Read the model definition and answer for the solid it produces. Units are mm, in the model's axes. A direction names the side the tool comes from. Round coordinates to 2 decimals unless told otherwise and drop trailing zeros. Loops run counter-clockwise (first coordinate to the right, second up) from the corner with the lowest first, then second, coordinate; pieces in that order, holes last. Notation, with made-up numbers: M 63.25,72 L 72.25,72 A21 ccw 72.25,91 Z; hole C 75.25,-36.5 d7. An arc over 180 degrees is marked long. Write each question's results on one line, items separated by ' | '.
from build123d import *

# Parameters (mm, degrees)
SKETCH1_R             = 1.5
BOSS_EXTRUDE1_DEPTH   = 5
BOSS_EXTRUDE1_2_DEPTH = 5
SKETCH1_3_R           = 5.25
BOSS_EXTRUDE2_DEPTH   = 2.5
SKETCH1_4_R           = 3.25
BOSS_EXTRUDE3_DEPTH   = 5
CUT_EXTRUDE1_DEPTH    = 34.791042337
CUT_EXTRUDE2_DEPTH    = 34.791042337
LPATTERN1_COUNT       = 28
LPATTERN1_PITCH       = 0.5
CUT_EXTRUDE3_DEPTH    = 34.791042337
CIRPATTERN1_COUNT     = 8
CIRPATTERN1_ANGLE     = 42


with BuildPart() as part:
    # Sketch1 → Boss-Extrude1 (new body)
    with BuildSketch(Plane.XY):
        with BuildLine():
            Line((-1.559459186, 5.819980914), (-9.630372069, 7.89024295))
            ThreePointArc((-9.630372069, 7.89024295), (-13.619847961, 6.086363356), (-12.727105745, 1.8))
            Line((-12.727105745, 1.8), (-9, 1.8))
            Line((-9, 1.8), (-9, 0))
            Line((-9, 0), (-5.25, 0))
            ThreePointArc((-5.25, 0), (-4.165105037, 3.195997502), (-1.358799987, 5.071110588))
            Line((-1.358799987, 5.071110588), (-1.559459186, 5.819980914))
        make_face()
        with Locations((-10.5, 4.5)):
            Circle(SKETCH1_R, mode=Mode.SUBTRACT)
    extrude(amount=BOSS_EXTRUDE1_DEPTH)



with BuildPart() as body_2:
    # Sketch1 → Boss-Extrude1 2 (new body)
    with BuildSketch(Plane.XY):
        with BuildLine():
            Line((5.983025461, -0.728942102), (5.162088265, 0.956736509))
            ThreePointArc((5.162088265, 0.956736509), (4.867715236, -1.966684615), (3.048690517, -4.274106471))
            Line((3.048690517, -4.274106471), (3.844408913, -5.389662519))
            Line((3.844408913, -5.389662519), (13.676957988, -3.567307264))
            Line((13.676957988, -3.567307264), (32.08570782, 4.250488438))
            Line((32.08570782, 4.250488438), (32.44741195, 6.013772341))
            Line((32.44741195, 6.013772341), (18.681843244, 3.462474984))
            ThreePointArc((18.681843244, 3.462474984), (14.653100202, 0.834635979), (9.916045092, 0))
            Line((9.916045092, 0), (5.983025461, -0.728942102))
        make_face()
    extrude(amount=BOSS_EXTRUDE1_2_DEPTH)


with BuildPart() as part_1:
    add(part.part)

    add(body_2.part)  # Boss-Extrude2 merges body 2
    # Sketch1<3> → Boss-Extrude2 (add)
    with BuildSketch(Plane.XY):
        Circle(SKETCH1_3_R)
    extrude(amount=BOSS_EXTRUDE2_DEPTH)

    # Sketch1<4> → Boss-Extrude3 (add)
    with BuildSketch(Plane.XY):
        Circle(SKETCH1_4_R)
    extrude(amount=BOSS_EXTRUDE3_DEPTH)

    # Sketch2 → Cut-Extrude1 (cut, through all)
    with BuildSketch(Plane(origin=(0, 0, 0), x_dir=(0.9832549075639557, 0.18223552549214142, 0), z_dir=(-0.18223552549214142, 0.9832549075639557, 0))):
        Polygon((13, 0), (33, -1.875), (33, 0), align=None)
        Polygon((33, -3.125), (33, -5), (13, -5), align=None)
    extrude(amount=-CUT_EXTRUDE1_DEPTH, mode=Mode.SUBTRACT)

    # Sketch3 → Cut-Extrude2 (cut, symmetric)
    with BuildSketch(Plane.XY):
        Polygon((31.759133514, 5.886207473), (32.03228257, 5.784278119), (32.250760968, 5.977325236), align=None)
    cut_extrude2 = extrude(amount=CUT_EXTRUDE2_DEPTH, both=True, mode=Mode.SUBTRACT)

    # LPattern1: Cut-Extrude2 ×28
    with Locations(*[Vector(-0.983254907563956, -0.1822355254921403, 0) * (i * LPATTERN1_PITCH) for i in range(1, LPATTERN1_COUNT)]):
        add(cut_extrude2, mode=Mode.SUBTRACT)

    # Sketch4 → Cut-Extrude3 (cut, through all)
    with BuildSketch(Plane.XY):
        Polygon((9.916045092, 0), (11.165663009, 0.030904073), (10.553215679, -0.48439513), align=None)
    cut_extrude3 = extrude(amount=CUT_EXTRUDE3_DEPTH, mode=Mode.SUBTRACT)

    # CirPattern1: Cut-Extrude3 ×8 about axis
    cirpattern1_axis = Axis((10.244577616, 11.995501923, 0), (0, 0, 1))
    for i in range(1, CIRPATTERN1_COUNT):
        add(cut_extrude3.rotate(cirpattern1_axis, i * CIRPATTERN1_ANGLE / (CIRPATTERN1_COUNT - 1)), mode=Mode.SUBTRACT)


solid = part_1.part
Item 1: Straight lines are drawn through the part: line 1 (Y direction, x = -10.5, z = 2.9); line 2 (X direction, y = 2.5, z = 3.15); line 3 (Z direction, x = 3.5, y = 3). For each, find the intervals that lie inside material, in ascending order.
Outcome:
line 1: y = 1.8 to 3, 6 to 8 | line 2: x = -13.37 to -4.62, -2.08 to 2.08, 17.93 to 27.96 | line 3: z = 0 to 2.5
Item 2: The part is cut by section A-A (x = -10.5). Determine the outline of the cut face in (y, z).
Outcome:
outline: M 1.8,0 L 3,0 L 3,5 L 1.8,5 Z; M 6,0 L 8,0 L 8,5 L 6,5 Z
Item 3: For faces 1 (the face through (3.44, -4.82, 2.46)), 2 (the face through (-0.1, -3.4, 2.5)), 3 (the face through (-11, 1.8, 2)), 4 (the face through (5.58, 0.1, 2.46)), determine the directions among +Z, -Z, +X, -X, +Y, -Y from which every point of the face is accessible in a straight line to the end or side of a thin tool.
Outcome:
face 1: +Z, -Z, -Y | face 2: +Z | face 3: +Z, -Z, -X, -Y | face 4: +Z, -Z, +Y
Item 4: The mould has two halves that part along X. Classify faces 5 (the face through (0, 0, 5)), 6 (the face through (20.71, -0.58, 2.46)), 7 (the face through (-12, 4.57, 2.46)): pulls with the +X half, pulls with the -X half, needs draft (parallel to the pull), parting line crosses it, or undercut.
Outcome:
face 5: needs draft | face 6: pulls with the +X half | face 7: undercut
Item 5: The part is cut by section B-B (x = 0). Determine the outline of the cut face in (y, z).
Outcome:
outline: M -5.25,0 L 5.25,0 L 5.25,2.5 L 3.25,2.5 L 3.25,5 L -3.25,5 L -3.25,2.5 L -5.25,2.5 Z
Item 6: The part is cut by section C-C (y = -1.25). Determine the outline of the cut face in (x, z).
Outcome:
outline: M -5.1,0 L 13.45,0 L 19.13,0.52 L 19.13,4.48 L 13.45,5 L 5.1,5 L 5.1,2.5 L 3,2.5 L 3,5 L -3,5 L -3,2.5 L -5.1,2.5 Z
Item 7: The part is cut by section D-D (x = 7). Determine the outline of the cut face in (y, z), plus the area to 3 significant figures.
Outcome:
outline: M -4.8,0 L -0.54,0 L -0.54,5 L -4.8,5 Z | area: 21.3 mm2
Item 8: Flat-ended cylindrical pins translate along their axes: pin 1 (1.5 mm diameter, centred on y = -4, z = 3.5, fed in from +X); pin 2 (2 mm diameter, centred on x = 8, z = 4, fed in from +Y); pin 3 (1.4 mm diameter, centred on y = 1, z = 3.5, fed in from -X). Find the tip coordinate at first contact, or state that the pin passes through.
Outcome:
pin 1: stops at x = 14.42 | pin 2: stops at y = -0.17 | pin 3: stops at x = -9
